```python
from build123d import *

# Parameters (mm, degrees)
SALIENTE_EXTRUIR1_DEPTH    = 30
CROQUIS2_R                 = 7.5
CORTAR_EXTRUIR1_DEPTH      = 4
CROQUIS3_R                 = 4.25
CORTAR_EXTRUIR2_DEPTH      = 16
CORTAR_EXTRUIR2_DEPTH_BACK = 16
CROQUIS5_R                 = 1.75
CORTAR_EXTRUIR3_DEPTH      = 1
CORTAR_EXTRUIR3_DEPTH_BACK = 22.73
CHAFL_N1_SIZE              = 0.5


with BuildPart() as part:
    # Croquis1 → Saliente-Extruir1 (new body)
    with BuildSketch(Plane.XY):
        with BuildLine():
            Line((-15.2, 0), (-8.7, 0))
            Line((-8.7, 0), (-5.415, 4.5))
            Line((-5.415, 4.5), (5.415, 4.5))
            Line((5.415, 4.5), (8.7, 0))
            Line((8.7, 0), (15.2, 0))
            ThreePointArc((15.2, 0), (15.553553391, -0.146446609), (15.7, -0.5))
            Line((15.7, -0.5), (15.7, -9.5))
            Line((15.7, -9.5), (16.75, -11.23))
            Line((16.75, -11.23), (16.75, -16.73))
            ThreePointArc((16.75, -16.73), (16.603553391, -17.083553391), (16.25, -17.23))
            Line((16.25, -17.23), (7.5, -17.23))
            Line((7.5, -17.23), (6, -16.23))
            Line((6, -16.23), (-6, -16.23))
            Line((-6, -16.23), (-7.5, -17.23))
            Line((-7.5, -17.23), (-16.25, -17.23))
            ThreePointArc((-16.25, -17.23), (-16.603553391, -17.083553391), (-16.75, -16.73))
            Line((-16.75, -16.73), (-16.75, -11.23))
            Line((-16.75, -11.23), (-15.7, -9.5))
            Line((-15.7, -9.5), (-15.7, -0.5))
            ThreePointArc((-15.7, -0.5), (-15.553553391, -0.146446609), (-15.2, 0))
        make_face()
    extrude(amount=SALIENTE_EXTRUIR1_DEPTH)

    # Croquis2 → Cortar-Extruir1 (cut)
    with BuildSketch(Plane.XY):
        with Locations((0, -5.5)):
            Circle(CROQUIS2_R)
    cortar_extruir1 = extrude(amount=CORTAR_EXTRUIR1_DEPTH, mode=Mode.SUBTRACT)

    # Simetría1: Cortar-Extruir1 across plane
    add(cortar_extruir1.mirror(Plane(origin=(0, 0, 15), x_dir=(1, 0, 0), z_dir=(0, 0, -1))), mode=Mode.SUBTRACT)

    # Croquis3 → Cortar-Extruir2 (cut, two sides)
    with BuildSketch(Plane(origin=(0, 0, 15), x_dir=(-1, 0, 0), z_dir=(0, 0, -1))) as cortar_extruir2_sk:
        with Locations((0, -5.5)):
            Circle(CROQUIS3_R)
    extrude(amount=CORTAR_EXTRUIR2_DEPTH, mode=Mode.SUBTRACT)
    extrude(cortar_extruir2_sk.sketch, amount=-CORTAR_EXTRUIR2_DEPTH_BACK, mode=Mode.SUBTRACT)

    # Croquis5 → Cortar-Extruir3 (cut, two sides)
    with BuildSketch(Plane.XZ.offset(17.23)) as cortar_extruir3_sk:
        with Locations((-11.8, 24.25)):
            Circle(CROQUIS5_R)
        with Locations((11.8, 24.25)):
            Circle(CROQUIS5_R)
        with Locations((11.8, 5.75)):
            Circle(CROQUIS5_R)
        with Locations((-11.8, 5.75)):
            Circle(CROQUIS5_R)
    extrude(amount=CORTAR_EXTRUIR3_DEPTH, mode=Mode.SUBTRACT)
    extrude(cortar_extruir3_sk.sketch, amount=-CORTAR_EXTRUIR3_DEPTH_BACK, mode=Mode.SUBTRACT)

    # Chaflán1
    chafl_n1_edges = [part.edges().sort_by_distance(p)[0] for p in [
        (-13.55, -17.23, 5.75),
        (10.05, -17.23, 5.75),
        (10.05, -17.23, 24.25),
        (-13.55, -17.23, 24.25),
    ]]
    chamfer(chafl_n1_edges, length=CHAFL_N1_SIZE)


solid = part.part
```
Geometry: final body of the model. Coordinates: model frame, mm. A direction names the side the tool comes from. Round coordinates to 2 decimals unless told otherwise and drop trailing zeros. Write each loop counter-clockwise with the first axis right and the second up, starting at its lowest first coordinate (ties: lowest second). Pieces come first, ordered by that corner, then holes.
Item 1: Section query C-C (x = 11.8). Return loops of the section in (y, z).
Item 2: Section query D-D (x = 0). Return loops of the section in (y, z), plus the area to 3 significant figures.
Item 3: Mould query, pull axis X, two halves, no side actions, for faces 4 (the face through (11.572, -8.482, 25.985)), 5 (the face through (3, -9, 26)), 6 (the face through (7.035, 2.282, 14.79)), 7 (the face through (-12, 0, 15)). Classes: +X half, -X half, draft (parallel to the pull), parting line (faces both ways), or undercut.
Item 4: Section query A-A (z = 5.75). Give the number of separate pieces and of enclosed holes in the cut face, plus the area to 3 significant figures.
Item 5: Pin query (flat end, axial travel): P1, Ø10, axis at y = -6, z = 16.5, coming from the -X side; P2, Ø3, axis at x = 11.8, z = 5.75, coming from the -Y side; P3, Ø1.5, axis at x = 4, y = -1, coming from the +Z side; P4, Ø10, axis at y = -5, z = 23, coming from the -X side. Return the tip coordinate at first contact, or that it passes through.
Item 6: Set-up query: faces 1 (the face through (3, -9, 4)), 2 (the face through (-6.74, -16.723, 14.79)), 3 (the face through (12, 0, 15)). Return all of +Z, -Z, +X, -X, +Y, -Y with unobstructed straight access to the full face (end or side cutting, diameter ignored); none if empty.
Item 7: Section query B-B (y = -5.5). Return loops of the section in (x, z), plus the area to 3 significant figures.
Item 8: Material intervals for L1, parallel to Z at x = 11.8, y = -12.5; L2, parallel to Y at x = 0, z = 7.5; L3, parallel to X at y = -5.5, z = 7, sorted ascending.
Completed:
1. outline: (-17.23, 0) - (0, 0) - (0, 4) - (-16.73, 4) - (-17.23, 3.5) - close; (-17.23, 8) - (-16.73, 7.5) - (0, 7.5) - (0, 22.5) - (-16.73, 22.5) - (-17.23, 22) - close; (-17.23, 26.5) - (-16.73, 26) - (0, 26) - (0, 30) - (-17.23, 30) - close
2. outline: (-16.23, 0) - (-13, 0) - (-13, 4) - (-9.75, 4) - (-9.75, 26) - (-13, 26) - (-13, 30) - (-16.23, 30) - close; (-1.25, 4) - (2, 4) - (2, 0) - (4.5, 0) - (4.5, 30) - (2, 30) - (2, 26) - (-1.25, 26) - close
2. area: 315 mm2
3. face 4: undercut
3. face 5: undercut
3. face 6: +X half
3. face 7: draft
4. separate pieces: 3
4. enclosed holes: 1
4. area: 427 mm2
5. P1: stops at x = -16.61
5. P2: passes through
5. P3: stops at z = 26
5. P4: stops at x = -16
6. face 1: -Z
6. face 2: +Z, -Z, -Y
6. face 3: +Z, -Z, +X, +Y
7. outline: (-15.7, 0) - (-7.5, 0) - (-7.5, 4) - (-4.25, 4) - (-4.25, 26) - (-7.5, 26) - (-7.5, 30) - (-15.7, 30) - close; (4.25, 4) - (7.5, 4) - (7.5, 0) - (15.7, 0) - (15.7, 30) - (7.5, 30) - (7.5, 26) - (4.25, 26) - close; hole circle Ø3.5 at (-11.8, 5.75); hole circle Ø3.5 at (-11.8, 24.25); hole circle Ø3.5 at (11.8, 5.75); hole circle Ø3.5 at (11.8, 24.25)
7. area: 597 mm2
8. L1: z = 0 to 4, 7.5 to 22.5, 26 to 30
8. L2: y = -16.23 to -9.75, -1.25 to 4.5
8. L3: x = -15.7 to -13.02, -10.58 to -4.25, 4.25 to 10.58, 13.02 to 15.7
